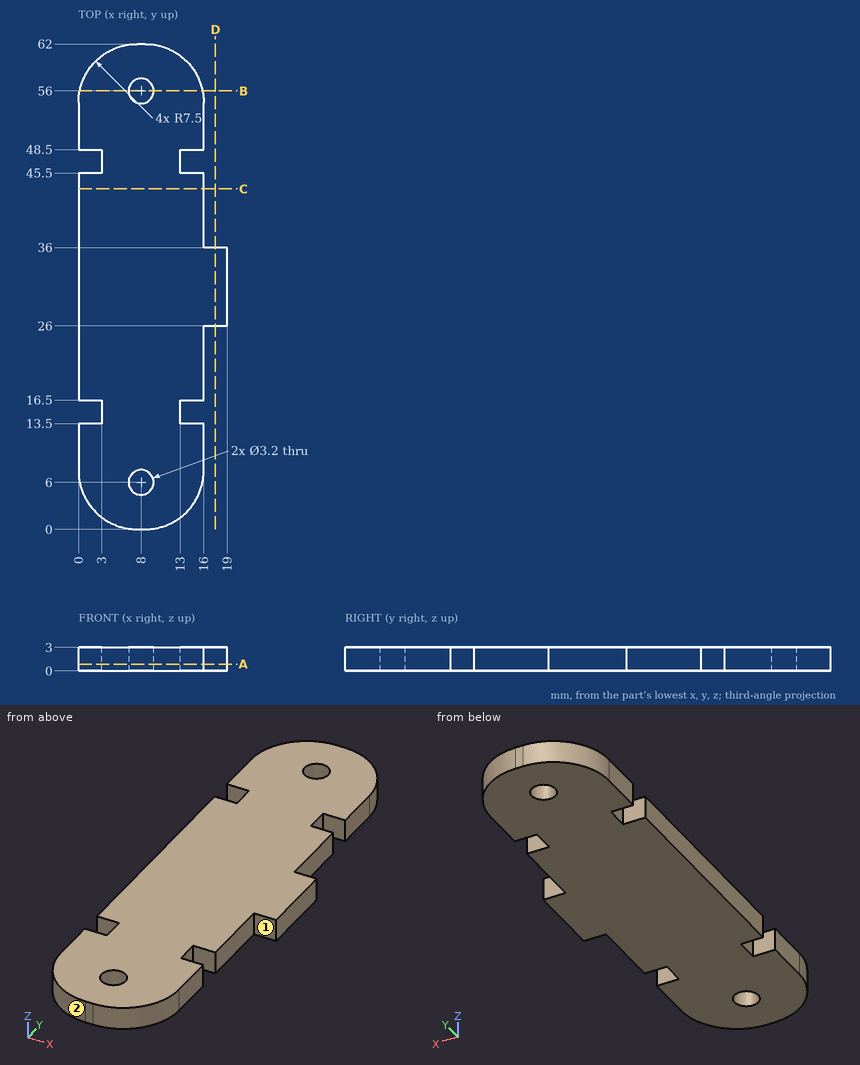
Geometry: see drawing. Coordinates: mm, zero at the bounding-box minimum. A direction names the side the tool comes from. Round coordinates to 2 decimals unless told otherwise and drop trailing zeros. Loops run counter-clockwise (first coordinate to the right, second up) from the corner with the lowest first, then second, coordinate; pieces in that order, holes last. Notation, with made-up numbers: (-3, -19.75) -> (12, -19.75) arc R11 cw to (12, -13.75) -> close; hole circle Ø7 at (77, -26.5). An arc over 180 degrees is marked (long way). Write each question's results on one line, items separated by ' | '.
1. Section C-C (y = 43.5). Return loops of the section in (x, z), and give its area (3 significant figures).
Geometry results:
outline: (0, 0) -> (16, 0) -> (16, 3) -> (0, 3) -> close | area: 48.0 mm2
2. Section A-A (z = 0.85). State how many separate pieces and enclosed holes the cut face has, and give its area (3 significant figures).
Geometry results:
separate pieces: 1 | enclosed holes: 2 | area: 922 mm2
3. Section D-D (x = 17.5). Return loops of the section in (y, z), and give its area (3 significant figures).
Geometry results:
outline: (26, 0) -> (36, 0) -> (36, 3) -> (26, 3) -> close | area: 30.0 mm2
4. Section B-B (y = 56). Return loops of the section in (x, z).
Geometry results:
outline: (0.15, 0) -> (6.4, 0) -> (6.4, 3) -> (0.15, 3) -> close; (9.6, 0) -> (15.85, 0) -> (15.85, 3) -> (9.6, 3) -> close
5. Ray query, line 1 (Y direction, x = 8, z = 1.45); line 2 (Y direction, x = 7.5, z = 0.55); line 3 (Y direction, x = 17, z = 1.7). Return the intervals inside material, ascending. Write a range as from..to.
Geometry results:
line 1: 0..4.4, 7.6..54.4, 57.6..62 | line 2: 0..4.48, 7.52..54.48, 57.52..62 | line 3: 26..36
6. First-contact query: P1, Ø1.5, axis at y = 15, z = 1.5, coming from the +X side; P2, Ø1.5, axis at x = 1.5, z = 1, coming from the +Y side; P3, Ø1.5, axis at y = 11.5, z = 1.5, coming from the +X side. Flat tips, straight axial feed; report the tip coordinate or a pass-through.
Geometry results:
P1: x = 13 | P2: y = 59.86 | P3: x = 16
7. Set-up query: the marked faces 1 and 2. Return all of +Z, -Z, +X, -X, +Y, -Y with unobstructed straight access to the full face (end or side cutting, diameter ignored); none if empty.
Geometry results:
face 1: +Z, -Z, +X, -Y | face 2: +Z, -Z, -X, -Y
